Could you check a few things on this model? Use its own coordinates, in mm. Give positions to 0.01 mm unless a question says otherwise; leave off trailing zeros. Loops run counter-clockwise (first coordinate to the right, second up) from the corner with the lowest first, then second, coordinate; pieces in that order, holes last. Notation, with made-up numbers: (33, -9.5) - (40, -9.5) arc R7 ccw to (40, 2.5) - close; hole circle Ø5 at (-40, 23). An arc over 180 degrees is marked (long way). Answer in a Markdown table with one row per item. Add a question column.
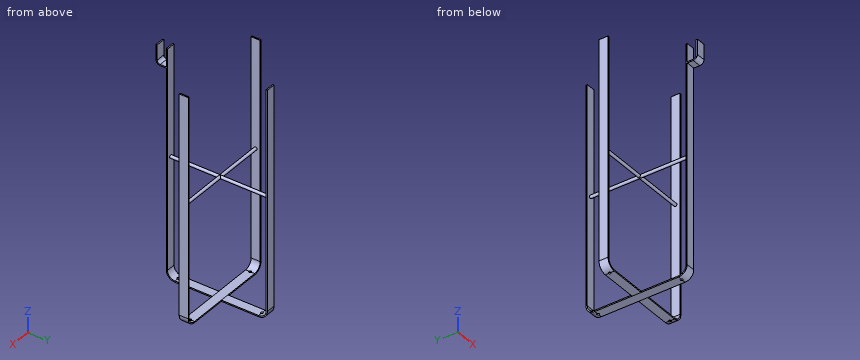
```python
from build123d import *

# Parameters (mm, degrees)
F1_DEPTH       = 30
F4_W           = 30
F4_H           = 4
F7_R           = 5
F8_DEPTH       = 334
F9_R           = 5
F10_DEPTH      = 334
F11_R          = 4
F12_DEPTH      = 25
F14_DEPTH      = 15
F14_DEPTH_BACK = 15


with BuildPart() as f1:
    # F0 (on Right) → F1 (new body)
    with BuildSketch(Plane.YZ):
        with BuildLine():
            Line((0, -725), (0, 0))
            Line((0, 0), (-4, 0))
            Line((-4, 0), (-4, -725))
            ThreePointArc((-4, -725), (4.4939033456, -745.5060966544), (25, -754))
            Line((25, -754), (302, -754))
            ThreePointArc((302, -754), (322.5060966544, -745.5060966544), (331, -725))
            Line((331, -725), (331, 0))
            Line((331, 0), (327, 0))
            Line((327, 0), (327, -725))
            ThreePointArc((327, -725), (319.6776695297, -742.6776695297), (302, -750))
            Line((302, -750), (25, -750))
            ThreePointArc((25, -750), (7.3223304703, -742.6776695297), (0, -725))
        make_face()
    extrude(amount=F1_DEPTH)

    # F6: sweep along a path in F5
    with BuildLine(Plane.XZ.offset(-148.5)) as f6_path:
        Line((-148.5, 0), (-148.5, -725))
        ThreePointArc((-148.5, -725), (-141.1776695297, -742.6776695297), (-123.5, -750))
        Line((-123.5, -750), (153.5, -750))
        ThreePointArc((153.5, -750), (171.1776695297, -742.6776695297), (178.5, -725))
        Line((178.5, -725), (178.5, 0))
    # F4 (on offset) → F6 (sweep)
    with BuildSketch(Plane.YZ.offset(15)):
        with Locations((163.5060608387, -751.9651731714)):
            Rectangle(F4_W, F4_H)
    sweep(path=f6_path.line)

    # F7 (on face) → F8 (join)
    with BuildSketch(Plane.YZ.offset(182.4651731714)):
        with Locations((163.5060608387, -360)):
            Circle(F7_R)
    extrude(amount=-F8_DEPTH)

    # F9 (on face) → F10 (join)
    with BuildSketch(Plane.XZ.offset(4)):
        with Locations((15, -360)):
            Circle(F9_R)
    extrude(amount=-F10_DEPTH)

    # F11 (on face) → F12 (cut)
    with BuildSketch(Plane(origin=(0, 0, -754), x_dir=(1, 0, 0), z_dir=(0, 0, -1))):
        with Locations((15, -25)):
            Circle(F11_R)
        with Locations((15, -302)):
            Circle(F11_R)
        with Locations((-123.1007874012, -163.7377291918)):
            Circle(F11_R)
        with Locations((154.1218459606, -164.2482578754)):
            Circle(F11_R)
    extrude(amount=-F12_DEPTH, mode=Mode.SUBTRACT)

    # F13 (on offset) → F14 (join, two sides)
    with BuildSketch(Plane.YZ.offset(15)) as f14_sk:
        with BuildLine():
            Line((-3.8402353227, -64), (-3.8402353227, -60))
            Line((-3.8402353227, -60), (-23.8402353227, -60))
            ThreePointArc((-23.8402353227, -60), (-30.9113031346, -57.0710678119), (-33.8402353227, -50))
            Line((-33.8402353227, -50), (-33.8402353227, 0))
            Line((-33.8402353227, 0), (-37.8402353227, 0))
            Line((-37.8402353227, 0), (-37.8402353227, -50))
            ThreePointArc((-37.8402353227, -50), (-33.7397302593, -59.8994949366), (-23.8402353227, -64))
            Line((-23.8402353227, -64), (-3.8402353227, -64))
        make_face()
    extrude(amount=F14_DEPTH)
    extrude(f14_sk.sketch, amount=-F14_DEPTH_BACK)


solid = f1.part
```
(1) I want a section at C-C on z = -430.5. Please give me the cut outline in (x, y).
(2) I want a section at B-B on y = 102. Please give me the cut outline in (x, z).
(3) For pin 1 Ø13 at (x, y) = (-123.1, 163.74) entering from -Z; pin 2 Ø9 at (x, y) = (18, 214.5) entering from +Z; pin 3 Ø2 at (y, z) = (181.5, -192.5) entering from -X, each with a flat end and sliding along its axis, tell me the tip position at first contact or that it passes through.
(4) I want a section at A-A on x = -57. Please give me the cut outline in (y, z), then the cut area to 3 significant figures.
(5) Please list where these lines run through material, in increasing order: line 1 (Y direction, x = 1, z = -402); line 2 (X direction, y = 302, z = -750.55); line 3 (Z direction, x = 20.5, y = 74).
Reported:
| question | item | result |
|---|---|---|
| 1 | outline | (-152.47, 148.51) - (-148.47, 148.51) - (-148.47, 178.51) - (-152.47, 178.51) - close; (0, -4) - (30, -4) - (30, 0) - (0, 0) - close; (0, 327) - (30, 327) - (30, 331) - (0, 331) - close; (178.47, 148.51) - (182.47, 148.51) - (182.47, 178.51) - (178.47, 178.51) - close |
| 2 | outline | (0, -754) - (30, -754) - (30, -750) - (0, -750) - close; circle Ø10 at (15, -360) |
| 3 | pin 1 | z = -753.97 |
| 3 | pin 2 | z = -355 |
| 3 | pin 3 | through |
| 4 | outline | (148.51, -753.97) - (178.51, -753.97) - (178.51, -749.97) - (148.51, -749.97) - close; circle Ø10 at (163.51, -360) |
| 4 | area | 199 mm² |
| 5 | line 1 | -4 to 0, 327 to 331 |
| 5 | line 2 | 0 to 11, 19 to 30 |
| 5 | line 3 | -754 to -750 |
